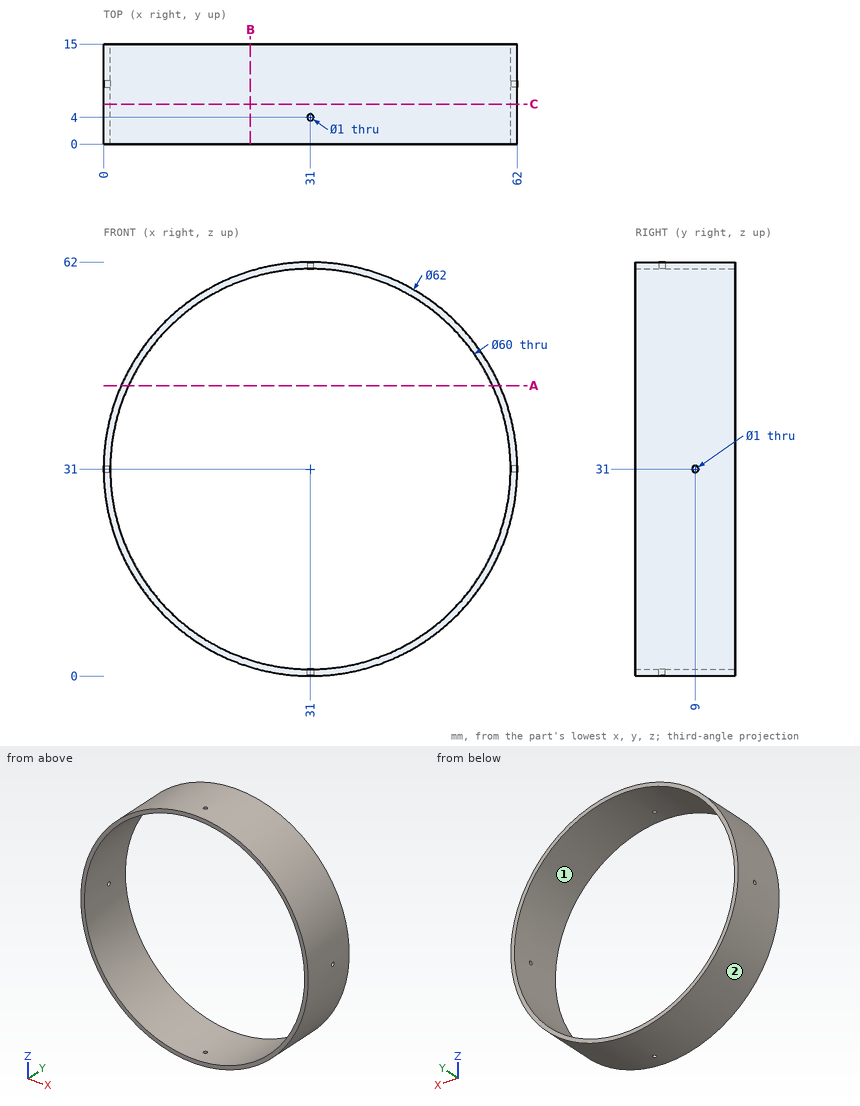
Geometry: see drawing. Coordinates: mm, zero at the bounding-box minimum. Round coordinates to 2 decimals unless told otherwise and drop trailing zeros. Loops run counter-clockwise (first coordinate to the right, second up) from the corner with the lowest first, then second, coordinate; pieces in that order, holes last. Notation, with made-up numbers: (32, 69.25) - (37, 69.25) arc R28 cw to (37, 107.25) - close; hole circle Ø7 at (85, 79.25). An arc over 180 degrees is marked (long way). One line per item, written item: value. Start each with the question number.
(1) Ray query, line 1 (X direction, y = 9.5, z = 33); line 2 (Z direction, x = 30.5, y = 5.25); line 3 (X direction, y = 13.75, z = 24). Return the intervals inside material, ascending. Write a range as [from, to].
(2) Contact query for flat-ended pins moving along their axis: P1, Ø2, axis at x = 32.5, y = 7, coming from the -Z side; P2, Ø2, axis at x = 45, y = 3.5, coming from the +Z side; P3, Ø4, axis at x = 9.5, y = 13, coming from the -Z side. Output: stop coordinate, or through.
(3) Section B-B, the plane x = 22. Return loops of the section in (y, z), plus the area to 3 significant figures.
(4) Draft query along Z for the marked faces 1 and 2. Return one class per face: +Z half, -Z half, draft (parallel to the pull), parting line (faces both ways), or undercut.
(5) Section C-C, the plane y = 6. Return loops of the section in (x, z), plus the area to 3 significant figures.
(6) Section A-A, the plane z = 43.5. Return loops of the section in (x, y).
Results below:
1. line 1: [0.06, 1.07], [60.93, 61.94]
1. line 2: [0, 1], [61, 62]
1. line 3: [0.8, 1.83], [60.17, 61.2]
2. P1: z = 0
2. P2: z = 59.14
2. P3: z = 6.9
3. outline: (0, 1.34) - (15, 1.34) - (15, 2.38) - (0, 2.38) - close; (0, 59.62) - (15, 59.62) - (15, 60.66) - (0, 60.66) - close
3. area: 31.4 mm^2
4. face 1: undercut
4. face 2: parting line
5. outline: circle Ø62 at (31, 31); hole circle Ø60 at (31, 31)
5. area: 192 mm^2
6. outline: (2.63, 0) - (3.73, 0) - (3.73, 15) - (2.63, 15) - close; (58.27, 0) - (59.37, 0) - (59.37, 15) - (58.27, 15) - close
